The model under review builds one solid part; all positions refer to its coordinate system, in mm. Give positions to 0.01 mm unless a question says otherwise; leave off trailing zeros. Write each loop counter-clockwise with the first axis right and the second up, starting at its lowest first coordinate (ties: lowest second). Pieces come first, ordered by that corner, then holes. Notation, with made-up numbers: (45.5, -22) -> (103.5, -22) arc R22 ccw to (103.5, -12) -> close; hole circle Ø11 at (21.25, 86.5). An arc over 180 degrees is marked (long way). Use CSV: the item, a comma, the result in double quotes.
```python
from build123d import *

# Parameters (mm, degrees)
SKETCH1_R                                 = 21.082
SKETCH1_R_2                               = 17.526
BOSS_EXTRUDE1_DEPTH                       = 1530.35
SKETCH4_W                                 = 3.373501
SKETCH4_H                                 = 21.082
F_17_64_0_26563_DIAMETER_HOLE1_AT_2_COUNT = 2
F_17_64_0_26563_DIAMETER_HOLE1_AT_2_PITCH = 1444.40656
F_17_64_0_26563_DIAMETER_HOLE2_D          = 6.747002


with BuildPart() as part:
    # Sketch1 → Boss-Extrude1 (new body)
    with BuildSketch(Plane(origin=(0, 0, 0), x_dir=(1, 0, 0), z_dir=(0, 1, 0))):
        with Locations(Location((0, 0, 0), (0, 0, 270))):
            Circle(SKETCH1_R)
        with Locations(Location((0, 0, 0), (0, 0, 270))):
            Circle(SKETCH1_R_2, mode=Mode.SUBTRACT)
    extrude(amount=BOSS_EXTRUDE1_DEPTH)

    # Sketch4 → 17/64 (0.26563) Diameter Hole1 (revolve, cut)
    with BuildSketch(Plane(origin=(0, 42.97172, 0), x_dir=(0, 1, 0), z_dir=(1, 0, 0))):
        with Locations((1.6867505, 10.541)):
            Rectangle(SKETCH4_W, SKETCH4_H)
    f_17_64_0_26563_diameter_hole1 = revolve(axis=Axis((0, 42.97172, -6.35), (0, 0, 1)), mode=Mode.SUBTRACT)

    # 17/64 (0.26563) Diameter Hole1 at 2: 17/64 (0.26563) Diameter Hole1 ×2
    with Locations(*[(0, i * F_17_64_0_26563_DIAMETER_HOLE1_AT_2_PITCH, 0) for i in range(1, F_17_64_0_26563_DIAMETER_HOLE1_AT_2_COUNT)]):
        add(f_17_64_0_26563_diameter_hole1, mode=Mode.SUBTRACT)

    # 17/64 (0.26563) Diameter Hole2 (through all)
    with Locations(Plane.XY):
        with Locations((0, 1487.37828), (0, 42.97172)):
            Hole(F_17_64_0_26563_DIAMETER_HOLE2_D / 2)


solid = part.part
```
Q1. Consider section B-B (y = 1047.5). Write out the cut boundary in (x, z).
Derived:
outline,"circle Ø42.16 at (0, 0); hole circle Ø35.05 at (0, 0)"
Q2. Consider section A-A (z = 0). Write out the cut boundary in (x, y), then the cut area to 3 significant figures.
Derived:
outline,"(-21.08, 0) -> (-17.53, 0) -> (-17.53, 1530.35) -> (-21.08, 1530.35) -> close; (17.53, 0) -> (21.08, 0) -> (21.08, 1530.35) -> (17.53, 1530.35) -> close"
area,"10,900 mm2"
Q3. Insertion check: pin 1 (8 mm diameter, centred on y = 499, z = -14, fed in from -X); pin 2 (12 mm diameter, centred on x = -9.5, z = 1, fed in from -Y); pin 3 (3 mm diameter, centred on y = 1103, z = -13, fed in from -X); pin 4 (4 mm diameter, centred on y = 1158.5, z = 3, fed in from +X). Each pin has a flat end and moves straight along its axis. Give the tip position at first contact, or say it passes through.
Derived:
pin 1,"stops at x = -18.56"
pin 2,"passes through"
pin 3,"stops at x = -17.67"
pin 4,"stops at x = 21.06"
Q4. The part is to be moulded in two halves that separate along X. For faces 1 (the cylindrical face through (-8.075, 754.463, 19.474)), 2 (the flat face through (16, 0, -8)), 3 (the cylindrical face through (-10.66, 754.46, -13.91)), say which applies: pulls with the +X half, pulls with the -X half, needs draft (parallel to the pull), parting line crosses it, or undercut.
Derived:
face 1,"parting line crosses it"
face 2,"needs draft"
face 3,"undercut"
Q5. To check wall thickness, follow probe 1 along Y at (x, z) = (0, 20.1); probe 2 along X at (y, z) = (235, -1.5); probe 3 along X at (y, z) = (528, 0). State the ranges of each line that lie inside material, in increasing order.
Derived:
probe 1,"y = 0 to 39.6, 46.35 to 1484, 1490.75 to 1530.35"
probe 2,"x = -21.03 to -17.46, 17.46 to 21.03"
probe 3,"x = -21.08 to -17.53, 17.53 to 21.08"
